Design review of the part built by this model. Coordinates are the model's own, in mm. Face numbers are marked on the shaded views. A direction names the side the tool comes from. Coordinates: 2 decimals unless noted, no trailing zeros. Write each loop counter-clockwise with the first axis right and the second up, starting at its lowest first coordinate (ties: lowest second). Pieces come first, ordered by that corner, then holes.
Q1. Take a section at C-C, the plane x = -82.5. Write out the cut boundary in (y, z).
Q2. Take a section at A-A, the plane x = -56.5. Write out the cut boundary in (y, z), plus the area to 3 significant figures.
Q3. For L1, parallel to Z at x = -82.5, y = 6; L2, parallel to X at y = 2.25, z = -27; L3, parallel to X at y = 5.9, z = -24, list the stretches that pass through material, from the lowest coordinate up.
Q4. The part is to be moulded in two halves that separate along Z. For the marked faces 3, 4 and 5, say which applies: released by +Z, released by -Z, zero draft, split by the parting line, or undercut.
Q5. For pin 1 Ø2 at (y, z) = (4.5, -22.5) entering from +X; pin 2 Ø1 at (y, z) = (5, -29) entering from +X, all flat-tipped, find the tip position at first contact; note any pin that passes through.
Q6. Take a section at B-B, the plane z = -24. Write out the cut boundary in (x, y), plus the area to 3 significant figures.
Q7. Take a section at D-D, the plane y = 5.5. Write out the cut boundary in (x, z), plus the area to 3 significant figures.
Q8. For the marked faces 1 and 2, list the 3-axis set-ups (+Z, -Z, +X, -X, +Y, -Y) from which the entire face can be reached by the end or side of a thin tool; tool diameter is ignored.
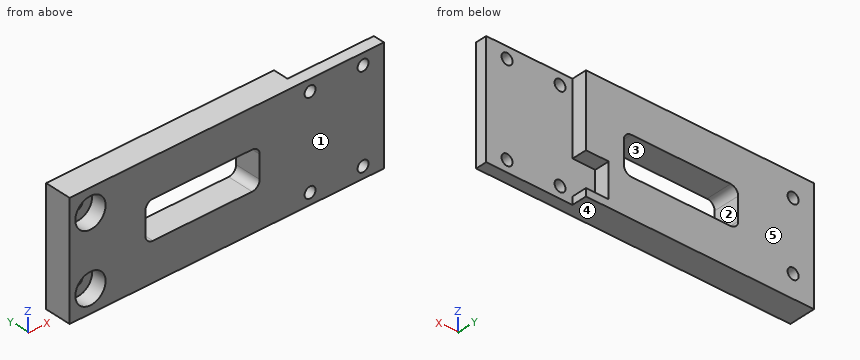
from build123d import *

# Parameters (mm, degrees)
SKETCH_1_W          = 88
SKETCH_1_H          = 30
EXTRUDE_1_DEPTH     = 3
SKETCH_2_W          = 27.8
SKETCH_2_H          = 30
CUT_EXTRUDE_1_DEPTH = 1
SKETCH_3_R          = 1.45
CUT_EXTRUDE_2_DEPTH = 11
SKETCH_4_R          = 1.45
CUT_EXTRUDE_4_DEPTH = 11
SKETCH_5_W          = 30.2
SKETCH_5_H          = 10
CUT_EXTRUDE_5_DEPTH = 11
FILLET_1_R          = 2
SKETCH_6_W          = 5
SKETCH_6_H          = 30
CUT_EXTRUDE_6_DEPTH = 10
SKETCH_9_W          = 60.2
SKETCH_9_H          = 30
SKETCH_9_R          = 1.45
EXTRUDE_4_DEPTH     = 4
EXTRUDE_START       = 1
SKETCH_7_W          = 22.8
SKETCH_7_H          = 30
SKETCH_7_R          = 1.45
EXTRUDE_5_DEPTH     = 1
SKETCH_11_W         = 15
SKETCH_11_H         = 4
CUT_EXTRUDE_8_DEPTH = 6
SKETCH_12_W         = 2
SKETCH_12_H         = 4
EXTRUDE_6_DEPTH     = 6
SKETCH_13_W         = 6
SKETCH_13_H         = 4
EXTRUDE_7_DEPTH     = 4
SKETCH_14_R         = 4
CUT_EXTRUDE_9_DEPTH = 4


with BuildPart() as part:
    # 草图1 → 凸台-拉伸1 (new body)
    with BuildSketch(Plane(origin=(0, 0, 0), x_dir=(1, 0, 0), z_dir=(0, 1, 0))):
        with Locations((-44, 15)):
            Rectangle(SKETCH_1_W, SKETCH_1_H)
    extrude(amount=EXTRUDE_1_DEPTH)

    # 草图2 → 切除-拉伸1 (cut)
    with BuildSketch(Plane(origin=(0, 3, 0), x_dir=(1, 0, 0), z_dir=(0, 1, 0))):
        with Locations((-13.9, 15)):
            Rectangle(SKETCH_2_W, SKETCH_2_H)
    extrude(amount=-CUT_EXTRUDE_1_DEPTH, mode=Mode.SUBTRACT)

    # 草图3 → 切除-拉伸2 (cut)
    with BuildSketch(Plane(origin=(0, 2, 0), x_dir=(1, 0, 0), z_dir=(0, 1, 0))):
        with Locations(Location((-24.5, 27, 0), (0, 0, 270))):
            Circle(SKETCH_3_R)
        with Locations(Location((-24.5, 3, 0), (0, 0, 270))):
            Circle(SKETCH_3_R)
        with Locations(Location((-10.5, 3, 0), (0, 0, 270))):
            Circle(SKETCH_3_R)
        with Locations(Location((-10.5, 27, 0), (0, 0, 270))):
            Circle(SKETCH_3_R)
    extrude(amount=-CUT_EXTRUDE_2_DEPTH, mode=Mode.SUBTRACT)

    # 草图4 → 切除-拉伸4 (cut)
    with BuildSketch(Plane(origin=(0, 3, 0), x_dir=(1, 0, 0), z_dir=(0, 1, 0))):
        with Locations(Location((-82.5, 24, 0), (0, 0, 270))):
            Circle(SKETCH_4_R)
        with Locations(Location((-82.5, 6, 0), (0, 0, 270))):
            Circle(SKETCH_4_R)
    extrude(amount=-CUT_EXTRUDE_4_DEPTH, mode=Mode.SUBTRACT)

    # 草图5 → 切除-拉伸5 (cut)
    with BuildSketch(Plane(origin=(0, 3, 0), x_dir=(1, 0, 0), z_dir=(0, 1, 0))):
        with Locations((-52.9, 15)):
            Rectangle(SKETCH_5_W, SKETCH_5_H)
    extrude(amount=-CUT_EXTRUDE_5_DEPTH, mode=Mode.SUBTRACT)

    # 圆角1
    fillet_1_edges = [part.edges().sort_by_distance(p)[0] for p in [
        (-68, 1.5, -10),
        (-68, 1.5, -20),
        (-37.8, 1.5, -20),
        (-37.8, 1.5, -10),
    ]]
    fillet(fillet_1_edges, radius=FILLET_1_R)

    # 草图6 → 切除-拉伸6 (cut)
    with BuildSketch(Plane.XZ):
        with Locations((-2.5, -15)):
            Rectangle(SKETCH_6_W, SKETCH_6_H)
    extrude(amount=-CUT_EXTRUDE_6_DEPTH, mode=Mode.SUBTRACT)

    # 草图9 → 凸台-拉伸4 (add)
    with BuildSketch(Plane(origin=(0, 3, 0), x_dir=(1, 0, 0), z_dir=(0, 1, 0))):
        with Locations((-57.9, 15)):
            Rectangle(SKETCH_9_W, SKETCH_9_H)
        with Locations(Location((-82.5, 6, 0), (0, 0, 270))):
            Circle(SKETCH_9_R, mode=Mode.SUBTRACT)
        with Locations(Location((-82.5, 24, 0), (0, 0, 270))):
            Circle(SKETCH_9_R, mode=Mode.SUBTRACT)
        with BuildLine():
            Line((-37.8, 12), (-37.8, 18))
            ThreePointArc((-37.8, 18), (-38.385786438, 19.414213562), (-39.8, 20))
            Line((-39.8, 20), (-66, 20))
            ThreePointArc((-66, 20), (-67.414213562, 19.414213562), (-68, 18))
            Line((-68, 18), (-68, 12))
            ThreePointArc((-68, 12), (-67.414213562, 10.585786438), (-66, 10))
            Line((-66, 10), (-39.8, 10))
            ThreePointArc((-39.8, 10), (-38.385786438, 10.585786438), (-37.8, 12))
        make_face(mode=Mode.SUBTRACT)
    extrude(amount=EXTRUDE_4_DEPTH)

    # 草图7 → 凸台-拉伸5 (add)
    with BuildSketch(Plane(origin=(0, 2, 0), x_dir=(1, 0, 0), z_dir=(0, 1, 0)).offset(EXTRUDE_START)):
        with Locations((-16.4, 15)):
            Rectangle(SKETCH_7_W, SKETCH_7_H)
        with Locations(Location((-10.5, 3, 0), (0, 0, 270))):
            Circle(SKETCH_7_R, mode=Mode.SUBTRACT)
        with Locations(Location((-24.5, 27, 0), (0, 0, 270))):
            Circle(SKETCH_7_R, mode=Mode.SUBTRACT)
        with Locations(Location((-10.5, 27, 0), (0, 0, 270))):
            Circle(SKETCH_7_R, mode=Mode.SUBTRACT)
        with Locations(Location((-24.5, 3, 0), (0, 0, 270))):
            Circle(SKETCH_7_R, mode=Mode.SUBTRACT)
    extrude(amount=-EXTRUDE_5_DEPTH)

    # 草图11 → 切除-拉伸8 (cut)
    with BuildSketch(Plane(origin=(-27.8, 0, 0), x_dir=(0, 0, -1), z_dir=(1, 0, 0))):
        with Locations((22.5, 5)):
            Rectangle(SKETCH_11_W, SKETCH_11_H)
    extrude(amount=-CUT_EXTRUDE_8_DEPTH, mode=Mode.SUBTRACT)

    # 草图12 → 凸台-拉伸6 (add)
    with BuildSketch(Plane(origin=(-33.8, 0, 0), x_dir=(0, 0, -1), z_dir=(1, 0, 0))):
        with Locations((29, 5)):
            Rectangle(SKETCH_12_W, SKETCH_12_H)
    extrude(amount=EXTRUDE_6_DEPTH)

    # 草图13 → 凸台-拉伸7 (add)
    with BuildSketch(Plane(origin=(0, 0, -15), x_dir=(-1, 0, 0), z_dir=(0, 0, -1))):
        with Locations((30.8, 5)):
            Rectangle(SKETCH_13_W, SKETCH_13_H)
    extrude(amount=EXTRUDE_7_DEPTH)

    # 草图14 → 切除-拉伸9 (cut)
    with BuildSketch(Plane.XZ):
        with Locations(Location((-82.5, -6, 0), (0, 0, 270))):
            Circle(SKETCH_14_R)
        with Locations(Location((-82.5, -24, 0), (0, 0, 270))):
            Circle(SKETCH_14_R)
    extrude(amount=-CUT_EXTRUDE_9_DEPTH, mode=Mode.SUBTRACT)


solid = part.part
Responses:
1. outline: (0, -30) - (7, -30) - (7, -25.45) - (4, -25.45) - (4, -28) - (0, -28) - close; (0, -20) - (4, -20) - (4, -22.55) - (7, -22.55) - (7, -7.45) - (4, -7.45) - (4, -10) - (0, -10) - close; (0, -2) - (4, -2) - (4, -4.55) - (7, -4.55) - (7, 0) - (0, 0) - close
2. outline: (0, -30) - (7, -30) - (7, -20) - (0, -20) - close; (0, -10) - (7, -10) - (7, 0) - (0, 0) - close
2. area: 140 mm2
3. L1: z = -30 to -25.45, -22.55 to -7.45, -4.55 to 0
3. L2: x = -88 to -85.15, -79.85 to -25.95, -23.05 to -11.95, -9.05 to -5
3. L3: x = -88 to -83.95, -81.05 to -33.8
4. face 3: undercut
4. face 4: released by -Z
4. face 5: zero draft
5. pin 1: stops at x = -33.8
5. pin 2: stops at x = -27.8
6. outline: (-88, 0) - (-86.5, 0) - (-86.5, 4) - (-83.95, 4) - (-83.95, 7) - (-88, 7) - close; (-81.05, 4) - (-78.5, 4) - (-78.5, 0) - (-5, 0) - (-5, 3) - (-33.8, 3) - (-33.8, 7) - (-81.05, 7) - close
6. area: 425 mm2
7. outline: (-88, -30) - (-27.8, -30) - (-27.8, -28) - (-33.8, -28) - (-33.8, -19) - (-27.8, -19) - (-27.8, 0) - (-88, 0) - close; hole circle Ø2.9 at (-82.5, -24); hole circle Ø2.9 at (-82.5, -6); hole (-68, -18) arc R2 ccw to (-66, -20) - (-39.8, -20) arc R2 ccw to (-37.8, -18) - (-37.8, -12) arc R2 ccw to (-39.8, -10) - (-66, -10) arc R2 ccw to (-68, -12) - close
7. area: 1,440 mm2
8. face 1: +Z, -Z, +X, -X, -Y
8. face 2: +Y, -Y
